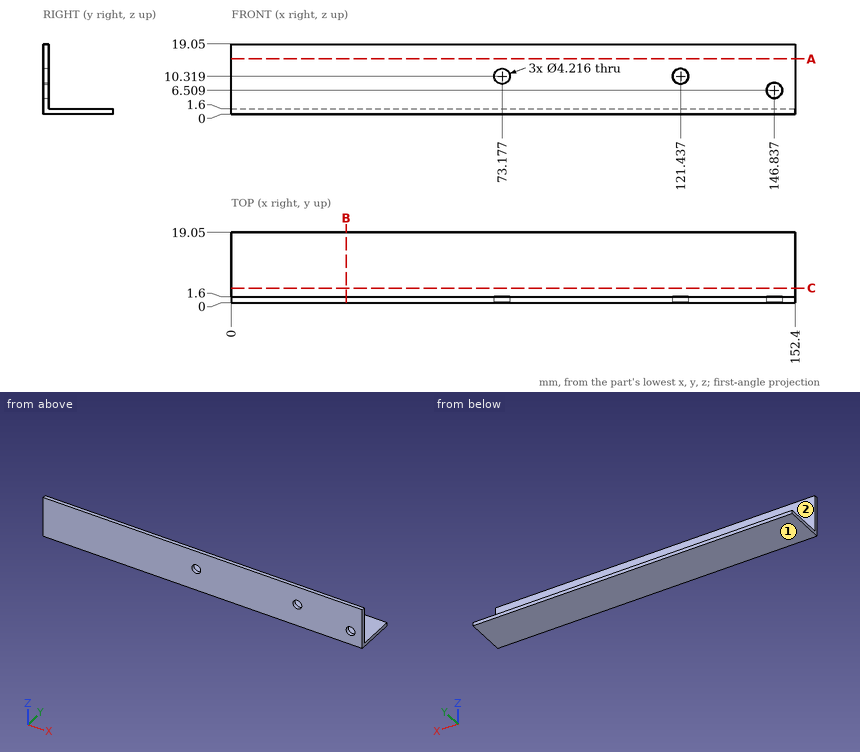
Drawing for the job (mm, zero at the part's lowest x, y, z). A direction names the side the tool comes from. Give positions to 0.01 mm unless a question says otherwise; leave off trailing zeros. Loops run counter-clockwise (first coordinate to the right, second up) from the corner with the lowest first, then second, coordinate; pieces in that order, holes last.
(1) Drill centre line: line 1 along Y through (x, z) = (116.5, 16.75). Where is it in solid material? Low to high.
Return value:
line 1: y = 0 to 1.6
(2) Band-saw the part on B-B (x = 31). Write the cut outline in (y, z).
Return value:
outline: (0, 0) - (19.05, 0) - (19.05, 1.6) - (1.6, 1.6) - (1.6, 19.05) - (0, 19.05) - close
(3) Pin check, flat tips, straight feed: pin 1 (1.5 mm diameter, centred on x = 63.5, y = 16.5, fed in from +Z); pin 2 (6.5 mm diameter, centred on x = 146.84, z = 6.51, fed in from +Y); pin 3 (4 mm diameter, centred on x = 73.18, z = 10.32, fed in from -Y). Stop position of each tip, or through.
Return value:
pin 1: stops at z = 1.6
pin 2: stops at y = 1.6
pin 3: passes through
(4) Band-saw the part on A-A (z = 15). Write the cut outline in (x, y), and give its area (3 significant figures).
Return value:
outline: (0, 0) - (152.4, 0) - (152.4, 1.6) - (0, 1.6) - close
area: 244 mm2
(5) 3-axis set-ups, long thin cutter, end or side, ignore diameter. For the marked faces 1 and 2: which of +Z, -Z, +X, -X, +Y, -Y reach the whole face in a straight line?
Return value:
face 1: -Z, +X, -X, +Y, -Y
face 2: +Z, +X, -X, +Y
